```python
from build123d import *

# Parameters (mm, degrees)
CROQUIS1_W              = 50
CROQUIS1_H              = 15
CROQUIS1_R              = 1.3
CROQUIS1_W_2            = 1.5
CROQUIS1_H_2            = 4
SALIENTE_EXTRUIR1_DEPTH = 2
CROQUIS2_R              = 1.5
SALIENTE_EXTRUIR2_DEPTH = 5
CHAFL_N1_SIZE           = 0.5
CHAFL_N2_SIZE           = 0.5


with BuildPart() as part:
    # Croquis1 → Saliente-Extruir1 (new body)
    with BuildSketch(Plane(origin=(0, 0, 0), x_dir=(1, 0, 0), z_dir=(0, 1, 0))):
        Rectangle(CROQUIS1_W, CROQUIS1_H)
        with Locations(Location((-16, 0, 0), (0, 0, 270))):
            Circle(CROQUIS1_R, mode=Mode.SUBTRACT)
        with Locations(Location((-7, 0, 0), (0, 0, 270))):
            Circle(CROQUIS1_R, mode=Mode.SUBTRACT)
        with Locations(Location((2, 0, 0), (0, 0, 270))):
            Circle(CROQUIS1_R, mode=Mode.SUBTRACT)
        with Locations(Location((11, 0, 0), (0, 0, 270))):
            Circle(CROQUIS1_R, mode=Mode.SUBTRACT)
        with Locations((18, 0)):
            Rectangle(CROQUIS1_W_2, CROQUIS1_H_2, mode=Mode.SUBTRACT)
    extrude(amount=SALIENTE_EXTRUIR1_DEPTH)

    # Croquis2 → Saliente-Extruir2 (add)
    with BuildSketch(Plane(origin=(0, 2, 0), x_dir=(1, 0, 0), z_dir=(0, 1, 0))):
        with Locations(Location((-22.5, 0, 0), (0, 0, 90))):
            Circle(CROQUIS2_R)
        with Locations(Location((22.5, 0, 0), (0, 0, 90))):
            Circle(CROQUIS2_R)
    extrude(amount=SALIENTE_EXTRUIR2_DEPTH)

    # Chaflán1
    chafl_n1_edges = [part.edges().sort_by_distance(p)[0] for p in [
        (-22.5, 7, 1.5),
    ]]
    chamfer(chafl_n1_edges, length=CHAFL_N1_SIZE)

    # Chaflán2
    chafl_n2_edges = [part.edges().sort_by_distance(p)[0] for p in [
        (22.5, 7, 1.5),
    ]]
    chamfer(chafl_n2_edges, length=CHAFL_N2_SIZE)


solid = part.part
```
Input: part model. Units: mm. Frame: model coordinates. A direction names the side the tool comes from. Round coordinates to 2 decimals unless told otherwise and drop trailing zeros. Loops run counter-clockwise (first coordinate to the right, second up) from the corner with the lowest first, then second, coordinate; pieces in that order, holes last. Notation, with made-up numbers: M 50,83.5 L 108,83.5 A16 cw 108,108.5 Z; hole C 13,-15 d1. An arc over 180 degrees is marked long. Answer in a Markdown table with one row per item. Add a question column.
1. Section B-B (x = -7). Output: boundary loops of the cut face in (y, z), and give its area (3 significant figures).
2. Set-up query: faces 5 (the face through (18, 1, 2)), 6 (the face through (21.235, 4.219, -0.806)), 7 (the face through (-25, 1, 0)). Return all of +Z, -Z, +X, -X, +Y, -Y with unobstructed straight access to the full face (end or side cutting, diameter ignored); none if empty.
3. Section A-A (y = 1). Output: boundary loops of the cut face in (x, z), and give its area (3 significant figures).
4. Contact query for flat-ended pins moving along their axis: pin 1 (4 mm diameter, centred on x = 11, z = 0, fed in from -Y); pin 2 (4 mm diameter, centred on y = 6, z = 4.5, fed in from -X); pin 3 (6 mm diameter, centred on x = -12.5, z = 4.5, fed in from +Y); pin 4 (2 mm diameter, centred on y = 5, z = 0, fed in from -X). Output: stop coordinate, or through.
5. Section C-C (x = -22.5). Output: boundary loops of the cut face in (y, z).
6. Ray query, probe 1 along X at (y, z) = (1.45, 0); probe 2 along Y at (x, z) = (-0.5, 0.25); probe 3 along X at (y, z) = (2.75, -1.25). Return the intervals inside material, ascending.
7. Section D-D (z = 0). Give the number of separate pieces and of enclosed holes in the cut face, and give its area (3 significant figures).
8. Mould query, pull axis Z, two halves, no side actions, for faces 1 (the face through (-24, 4, 0)), 2 (the face through (17.25, 1, 0)), 3 (the face through (25, 1, 0)), 4 (the face through (18, 1, -2)). Classes: released by +Z, released by -Z, zero draft, split by the parting line, or undercut.
Values follow:
| question | item | result |
|---|---|---|
| 1 | outline | M 0,-7.5 L 2,-7.5 L 2,-1.3 L 0,-1.3 Z; M 0,1.3 L 2,1.3 L 2,7.5 L 0,7.5 Z |
| 1 | area | 24.8 mm^2 |
| 2 | face 5 | +Y, -Y |
| 2 | face 6 | +Y |
| 2 | face 7 | +Z, -Z, -X, +Y, -Y |
| 3 | outline | M -25,-7.5 L 25,-7.5 L 25,7.5 L -25,7.5 Z; hole C -16,0 d2.6; hole C -7,0 d2.6; hole C 2,0 d2.6; hole C 11,0 d2.6; hole M 17.25,-2 L 18.75,-2 L 18.75,2 L 17.25,2 Z |
| 3 | area | 723 mm^2 |
| 4 | pin 1 | y = 0 |
| 4 | pin 2 | through |
| 4 | pin 3 | y = 2 |
| 4 | pin 4 | x = -24 |
| 5 | outline | M 0,-7.5 L 2,-7.5 L 2,-1.5 L 6.5,-1.5 L 7,-1 L 7,1 L 6.5,1.5 L 2,1.5 L 2,7.5 L 0,7.5 Z |
| 6 | probe 1 | -25 to -17.3, -14.7 to -8.3, -5.7 to 0.7, 3.3 to 9.7, 12.3 to 17.25, 18.75 to 25 |
| 6 | probe 2 | 0 to 2 |
| 6 | probe 3 | -23.33 to -21.67, 21.67 to 23.33 |
| 7 | separate pieces | 6 |
| 7 | enclosed holes | 0 |
| 7 | area | 106 mm^2 |
| 8 | face 1 | split by the parting line |
| 8 | face 2 | undercut |
| 8 | face 3 | zero draft |
| 8 | face 4 | undercut |
